Part model, mm, in its own coordinate system. A direction names the side the tool comes from. Round coordinates to 2 decimals unless told otherwise and drop trailing zeros. Write each loop counter-clockwise with the first axis right and the second up, starting at its lowest first coordinate (ties: lowest second). Pieces come first, ordered by that corner, then holes. Notation, with made-up numbers: (-3.75, -1.5) -> (0.25, -1.5) arc R35 cw to (0.25, 36.5) -> close; hole circle Ø6 at (-30.75, 43). An arc over 180 degrees is marked (long way). Return JSON: item names as keys, results as strings. Group by question number.
```python
from build123d import *

# Parameters (mm, degrees)
F0_R     = 63.5
F1_DEPTH = 12.7
F2_T     = -2.54
F3_R     = 1.5875
F4_DEPTH = 12.7


with BuildPart() as f1:
    # F0 (on Front) → F1 (new body)
    with BuildSketch(Plane.XZ):
        Circle(F0_R)
    extrude(amount=F1_DEPTH)

    # F2
    f2_openings = [f1.faces().sort_by_distance(p)[0] for p in [
        (0, -12.7, 0),
    ]]
    offset(amount=F2_T, openings=f2_openings)

    # F3 (on face) → F4 (join)
    with BuildSketch(Plane.XZ.offset(2.54)):
        Circle(F3_R)
    extrude(amount=F4_DEPTH)


solid = f1.part
```
Item 1: Cut at D-D (z = 40.5). Write the cut outline in (x, y), then the cut area to 3 significant figures.
Item 2: Cut at A-A (z = 0). Write the cut outline in (x, y), then the cut area to 3 significant figures.
Item 3: Which spindle directions (+Z, -Z, +X, -X, +Y, -Y) get a long thin tool onto all of the face, cutting with end or side? Do faces 1 (the face through (-1, 0, 1)), 2 (the face through (-0.34, -8.8, -1.55)). Say none if no direction does.
Item 4: Cut at C-C (x = 0). Write the cut outline in (y, z), then the cut area to 3 significant figures.
Item 5: Cut at B-B (y = -9.5). Write the cut outline in (x, z) (1 decimal).
Item 6: Two-plate mould, pull along Z, no slides. Class faces 3 (the face through (-13.77, -6.26, -61.99)), 4 (the face through (0, -15.24, 0)), 5 (the face through (-13.21, -7.55, -59.51)): released by +Z, released by -Z, zero draft, split by the parting line, or undercut.
Item 7: Wall check: L1, parallel to Z at x = 0, y = -6; L2, parallel to Y at x = 24, z = 0; L3, parallel to X at y = -4.5, z = 45. Give the ranges that are in metal, low to high.
Item 8: Flat gauge pins, fed straight in: P1, Ø4, axis at x = -50, y = -10, coming from the -Z side; P2, Ø1.5, axis at x = 12.5, y = -6, coming from the +Z side; P3, Ø3, axis at x = 41.5, y = -6.5, coming from the +Z side. Where does each tip first touch, or does it go through?
Checks:
{
 "1": {"outline": "(-48.91, -12.7) -> (-45.56, -12.7) -> (-45.56, -2.54) -> (45.56, -2.54) -> (45.56, -12.7) -> (48.91, -12.7) -> (48.91, 0) -> (-48.91, 0) -> close", "area": "316 mm2"},
 "2": {"outline": "(-63.5, -12.7) -> (-60.96, -12.7) -> (-60.96, -2.54) -> (-1.59, -2.54) -> (-1.59, -15.24) -> (1.59, -15.24) -> (1.59, -2.54) -> (60.96, -2.54) -> (60.96, -12.7) -> (63.5, -12.7) -> (63.5, 0) -> (-63.5, 0) -> close", "area": "415 mm2"},
 "3": {"face 1": "+Z, -Z, +X, -X, +Y", "face 2": "-Y"},
 "4": {"outline": "(-15.24, -1.59) -> (-2.54, -1.59) -> (-2.54, -60.96) -> (-12.7, -60.96) -> (-12.7, -63.5) -> (0, -63.5) -> (0, 63.5) -> (-12.7, 63.5) -> (-12.7, 60.96) -> (-2.54, 60.96) -> (-2.54, 1.59) -> (-15.24, 1.59) -> close", "area": "415 mm2"},
 "5": {"outline": "circle Ø127 at (0, 0); circle Ø3.2 at (0, 0); hole circle Ø121.9 at (0, 0)"},
 "6": {"face 3": "split by the parting line", "face 4": "zero draft", "face 5": "undercut"},
 "7": {"L1": "z = -63.5 to -60.96, -1.59 to 1.59, 60.96 to 63.5", "L2": "y = -2.54 to 0", "L3": "x = -44.8 to -41.12, 41.12 to 44.8"},
 "8": {"P1": "stops at z = -41.57", "P2": "stops at z = 62.4", "P3": "stops at z = 49.32"}
}
